```python
from build123d import *

# Parameters (mm, degrees)
BOSS_EXTRUDE1_DEPTH = 100


with BuildPart() as part:
    # Sketch1 → Boss-Extrude1 (new body)
    with BuildSketch(Plane(origin=(0, 0, 0), x_dir=(1, 0, 0), z_dir=(0, 1, 0))):
        Polygon((-146.64355653, -95.4), (146.64355653, -95.4), (146.64355653, -44.6), (25.4, 165.4), (12.7, 165.4), (12.7, 190.8), (31.75, 190.8), (31.75, 197.15), (-31.75, 197.15), (-31.75, 190.8), (-12.7, 190.8), (-12.7, 165.4), (-25.4, 165.4), (-146.64355653, -44.6), align=None)
        Polygon((25.4, 114.6), (95.84355653, -44.6), (-95.84355653, -44.6), (-25.4, 114.6), align=None, mode=Mode.SUBTRACT)
    extrude(amount=BOSS_EXTRUDE1_DEPTH)


solid = part.part
```
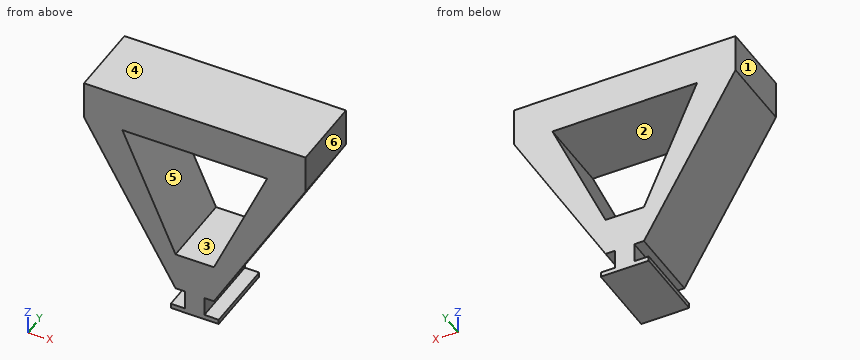
CAD build for the part. Positions are in the model's coordinates, mm. Face numbers are marked on the shaded views. A direction names the side the tool comes from. Round coordinates to 2 decimals unless told otherwise and drop trailing zeros. Write each loop counter-clockwise with the first axis right and the second up, starting at its lowest first coordinate (ties: lowest second). Pieces come first, ordered by that corner, then holes.
Item 1: Band-saw the part on A-A on x = -3.5. Write the cut outline in (y, z).
Filled in:
outline: (0, -197.15) - (100, -197.15) - (100, -114.6) - (0, -114.6) - close; (0, 44.6) - (100, 44.6) - (100, 95.4) - (0, 95.4) - close
Item 2: Band-saw the part on D-D on z = -160.5. Write the cut outline in (x, y), then the cut area to 3 significant figures.
Filled in:
outline: (-28.23, 0) - (28.23, 0) - (28.23, 100) - (-28.23, 100) - close
area: 5,650 mm2
Item 3: Tool access for the marked faces 1 and 2: list every direction of +Z, -Z, +X, -X, +Y, -Y with a clear straight run to the whole face (end or side of a thin tool).
Filled in:
face 1: +Z, -Z, -X, +Y, -Y
face 2: +Y, -Y
Item 4: Drop flat-ended pins along their axis: pin 1 Ø5 at (y, z) = (56, 32.5) entering from -X; pin 2 Ø1 at (x, y) = (80.5, 41.5) entering from -Z; pin 3 Ø20.5 at (y, z) = (33, -174) entering from -X. Give the stop position or say it passes through.
Filled in:
pin 1: stops at x = -141.1
pin 2: stops at z = -70.83
pin 3: stops at x = -26.35
Item 5: Drill centre lines: L1, parallel to Z at x = 16, y = 67; L2, parallel to Z at x = 27, y = 5.5; L3, parallel to X at y = 29.5, z = -167.5. Where is each one in solid material? Low to high.
Filled in:
L1: z = -197.15 to -190.8, -165.4 to -114.6, 44.6 to 95.4
L2: z = -197.15 to -190.8, -162.63 to -110.98, 44.6 to 95.4
L3: x = -12.7 to 12.7
Item 6: Band-saw the part on C-C on z = -72.5. Write the cut outline in (x, y), then the cut area to 3 significant figures.
Filled in:
outline: (-79.04, 0) - (-44.03, 0) - (-44.03, 100) - (-79.04, 100) - close; (44.03, 0) - (79.04, 0) - (79.04, 100) - (44.03, 100) - close
area: 7,000 mm2
Item 7: Mould opens along Z. For the marked faces 3, 4, 5 and 6 say: released by +Z, released by -Z, zero draft, split by the parting line, or undercut.
Filled in:
face 3: undercut
face 4: released by +Z
face 5: undercut
face 6: zero draft
Item 8: Band-saw the part on B-B on y = 63.5. Write the cut outline in (x, z).
Filled in:
outline: (-146.64, 44.6) - (-25.4, -165.4) - (-12.7, -165.4) - (-12.7, -190.8) - (-31.75, -190.8) - (-31.75, -197.15) - (31.75, -197.15) - (31.75, -190.8) - (12.7, -190.8) - (12.7, -165.4) - (25.4, -165.4) - (146.64, 44.6) - (146.64, 95.4) - (-146.64, 95.4) - close; hole (-95.84, 44.6) - (-25.4, -114.6) - (25.4, -114.6) - (95.84, 44.6) - close
